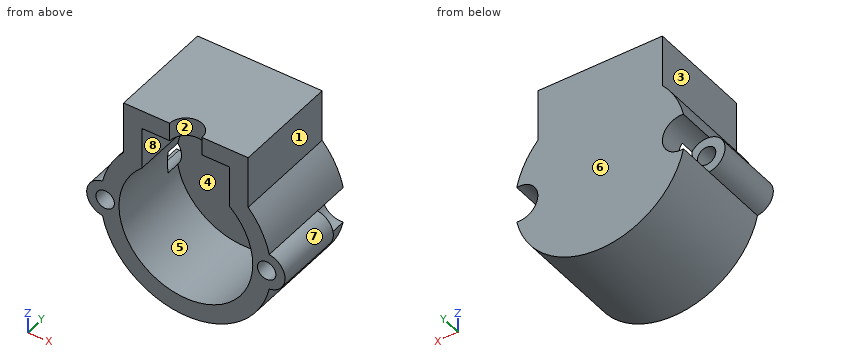
Autodesk Inventor part; units mm, degrees
ref_plane "YZ Plane" through (0, 0, 0) normal (1, 0, 0) x (0, 1, 0)
ref_plane "XZ Plane" through (0, 0, 0) normal (0, 1, 0) x (-1, 0, 0)
ref_plane "XY Plane" through (0, 0, 0) normal (0, 0, 1) x (1, 0, 0)
sketch "Sketch1" plane through (0, 0, 0) normal (0, 1, 0) x (-1, 0, 0)
  arc A0 (-9.5, 10.9545) -> (9.5, 10.9545) centre (0, 0) ccw
  line L0 (-9.5, 10.9545) -> (-9.5, 20)
  line L1 (-9.5, 20) -> (9.5, 20)
  line L2 (9.5, 20) -> (9.5, 10.9545)
  line L3 (13.5, 12.6491) -> (13.5, 24)
  line L4 (13.5, 24) -> (-13.5, 24)
  line L5 (-13.5, 24) -> (-13.5, 12.6491)
  arc A1 (-13.5, 12.6491) -> (13.5, 12.6491) centre (0, 0) ccw
  point P0 (0, -20)
  point P1 (-9.5, 15)
  dimension "d0" = 0
  dimension "d1" = 29
  dimension "d6" = 20
  dimension "d7" = 19
  dimension "d8" = 4
extrude "Extrusion1" add sketch "Sketch1" along normal blind 18
sketch "Sketch2" plane through (0, 18, 0) normal (0, 1, 0) x (1, 0, 0)
  arc A0 (13.5, -12.6491) -> (-13.5, -12.6491) centre (0, 0) ccw
  line L0 (-13.5, -12.6491) -> (-13.5, -24)
  line L1 (-13.5, -24) -> (13.5, -24)
  line L2 (13.5, -24) -> (13.5, -12.6491)
  line L3 (-13.5, -12.6491) -> (-13.5, -24)
extrude "Extrusion2" add sketch "Sketch2" along normal blind 5
sketch "Sketch3" plane through (-13.5, 0, 24) normal (0, 0, 1) x (1, 0, 0)
  circle A0 centre (13.5, 0) radius 3.5
  dimension "d13" = 7
extrude "Extrusion3" cut sketch "Sketch3" against normal blind 5
sketch "Sketch7" plane through (0, 0, 0) normal (0, -1, 0) x (1, 0, 0)
  circle A0 centre (-17.5, 0) radius 2
  circle A1 centre (17.5, 0) radius 2
  arc A2 (-18.0714, 3.959) -> (-18.0714, -3.959) centre (-17.5, 0) ccw
  arc A3 (18.0714, -3.959) -> (18.0714, 3.959) centre (17.5, 0) ccw
  arc A4 (-13.5, 12.6491) -> (13.5, 12.6491) centre (0, 0) ccw
  point P0 (18.4143, 1.7788)
  point P1 (18.4143, -1.7788)
  point P2 (-18.4143, -1.7788)
  point P3 (-18.4143, 1.7788)
  dimension "d29" = 4
  dimension "d30" = 4
  dimension "d31" = 35
  dimension "d32" = 17.5
  dimension "d33" = 8
  dimension "d34" = 8
extrude "Extrusion6" add sketch "Sketch7" against normal blind 15 contours A0 A4 A2 | A1 A4 A3
extrude "Extrusion7" cut sketch "Sketch7" against normal blind 15 contours A0 A4 | A4 A1 picked at (-17.4936, 0) picked at (17.4985, 0.08)
sketch "Sketch8" plane through (0, 0, 0) normal (0, 0, 1) x (1, 0, 0)
  line L0 (17.5, 15) -> (21.5, 15)
  line L1 (21.5, 15) -> (21.5, 19)
  line L2 (21.5, 19) -> (17.5, 19)
  line L3 (17.5, 19) -> (17.5, 15)
  line L4 (18.0714, 0) -> (-18.0714, 0)
  line L5 (21.5, 15) -> (18.0714, 15)
  point P0 (0, 0)
  point P1 (0, 0)
  dimension "d39" = 17.5
  dimension "d40" = 0
  dimension "d41" = 4
  dimension "d42" = 4
revolve "Revolution1" cut sketch "Sketch8" angle 360 about axis through (17.5, 19, 0) along (0, -1, 0)
sketch "Sketch9" plane through (17.5, 19, 0) normal (0, -1, 0) x (1, 0, 0)
  arc A0 (0.5714, 3.959) -> (0.5714, -3.959) centre (0, 0) ccw
  point P0 (-17.5, 0)
hole "Hole1" at (17.5, 19, 0) direction (0, 1, 0) diameter 8 end through all
mirror "Mirror1" about plane through (0, 0, 0) normal (1, 0, 0) of "Revolution1"
sketch "Sketch10" plane through (-17.5, 19, 0) normal (0, -1, 0) x (1, 0, 0)
  arc A0 (3.2, -2.4) -> (3.2, 2.4) centre (0, 0) ccw
  point P0 (17.5, 0)
hole "Hole2" at (-17.5, 19, 0) direction (0, 1, 0) diameter 8 end through all
properties part number "motor_holder_v2"
The model under review builds one solid part; all positions refer to its coordinate system, in mm. Face numbers are marked on the shaded views. A direction names the side the tool comes from. Round coordinates to 2 decimals unless told otherwise and drop trailing zeros. Order: outer loops, then holes, each group sorted by start corner. A loop starts at its lowest first (then second) coordinate and runs counter-clockwise, first axis right, second up. Notation, with made-up numbers: M 35,47.5 L 91,47.5 A6 cw 91,55.5 Z; hole C 2.25,13 d3. An arc over 180 degrees is marked long. Use a Markdown table: item, result.
1) Insertion check: pin 1 (10 mm diameter, centred on x = 3, y = 6.5, fed in from -Z); pin 2 (6 mm diameter, centred on x = -18, z = 1, fed in from +Y); pin 3 (9 mm diameter, centred on y = 11, z = 17, fed in from -X); pin 4 (7 mm diameter, centred on y = 10, z = 17, fed in from +X). Each pin has a flat end and moves straight along its axis. Give the tip position at first contact, or say it passes through.
Report:
| item | result |
|---|---|
| pin 1 | z = -18.5 |
| pin 2 | y = 23 |
| pin 3 | x = -13.64 |
| pin 4 | x = 13.5 |
2) Consider section A-A (z = 0). Write out the cut boundary in (x, y).
Report:
| item | result |
|---|---|
| outline | M -21.5,0 L -19.5,0 L -19.5,15 L -21.5,15 Z; M -15.5,0 L -14.5,0 L -14.5,15 L -15.5,15 Z; M -13.5,18 L 13.5,18 L 13.5,23 L -13.5,23 Z; M 14.5,0 L 15.5,0 L 15.5,15 L 14.5,15 Z; M 19.5,0 L 21.5,0 L 21.5,15 L 19.5,15 Z |
3) Consider section D-D (x = 0). Write out the cut boundary in (y, z), then the cut area to 4 significant figures.
Report:
| item | result |
|---|---|
| outline | M 0,-18.5 L 23,-18.5 L 23,24 L 3.5,24 L 3.5,20 L 18,20 L 18,-14.5 L 0,-14.5 Z |
| area | 342.5 mm^2 |
4) Wall thickness on line 1 along X through (y, z) = (15.25, 18); line 2 along Z through (x, y) = (7.5, 3.25); line 3 along X through (y, z) = (20, 0): over which ranges is each line inside the solid? List them lowest first. Write a range as [from, to].
Report:
| item | result |
|---|---|
| line 1 | [-13.5, -9.5], [9.5, 13.5] |
| line 2 | [-16.91, -12.41], [20, 24] |
| line 3 | [-13.5, 13.5] |
5) Draft analysis for pull direction X (two halves, no side actions). For the marked faces 5, 6, 7 and 8, state which applies: released by +X, released by -X, zero draft, split by the parting line, or undercut.
Report:
| item | result |
|---|---|
| face 5 | undercut |
| face 6 | zero draft |
| face 7 | released by +X |
| face 8 | undercut |
6) Consider section B-B (x = 17.5). Write out the cut boundary in (y, z).
Report:
| item | result |
|---|---|
| outline | M 0,-6 L 23,-6 L 23,-4 L 15,-4 L 15,-2 L 0,-2 Z; M 0,2 L 15,2 L 15,4 L 23,4 L 23,6 L 0,6 Z |
7) Consider section C-C (y = 4.25). Write out the cut boundary in (x, z).
Report:
| item | result |
|---|---|
| outline | M -18.07,-3.96 A18.5 ccw 18.07,-3.96 A4 ccw 18.07,3.96 A18.5 ccw 13.5,12.65 L 13.5,24 L -13.5,24 L -13.5,12.65 A18.5 ccw -18.07,3.96 A4 ccw Z; hole C -17.5,0 d4; hole M -9.5,10.95 A14.5 ccw long 9.5,10.95 L 9.5,20 L -9.5,20 Z; hole C 17.5,0 d4 |
8) Tool access review of the marked faces 1, 2, 3 and 4: name each direction out of +Z, -Z, +X, -X, +Y, -Y from which nothing blocks a thin tool from reaching the whole face with its end or side.
Report:
| item | result |
|---|---|
| face 1 | +Z, +X, +Y, -Y |
| face 2 | +Z, -Y |
| face 3 | +Z, -X, +Y, -Y |
| face 4 | -Y |
